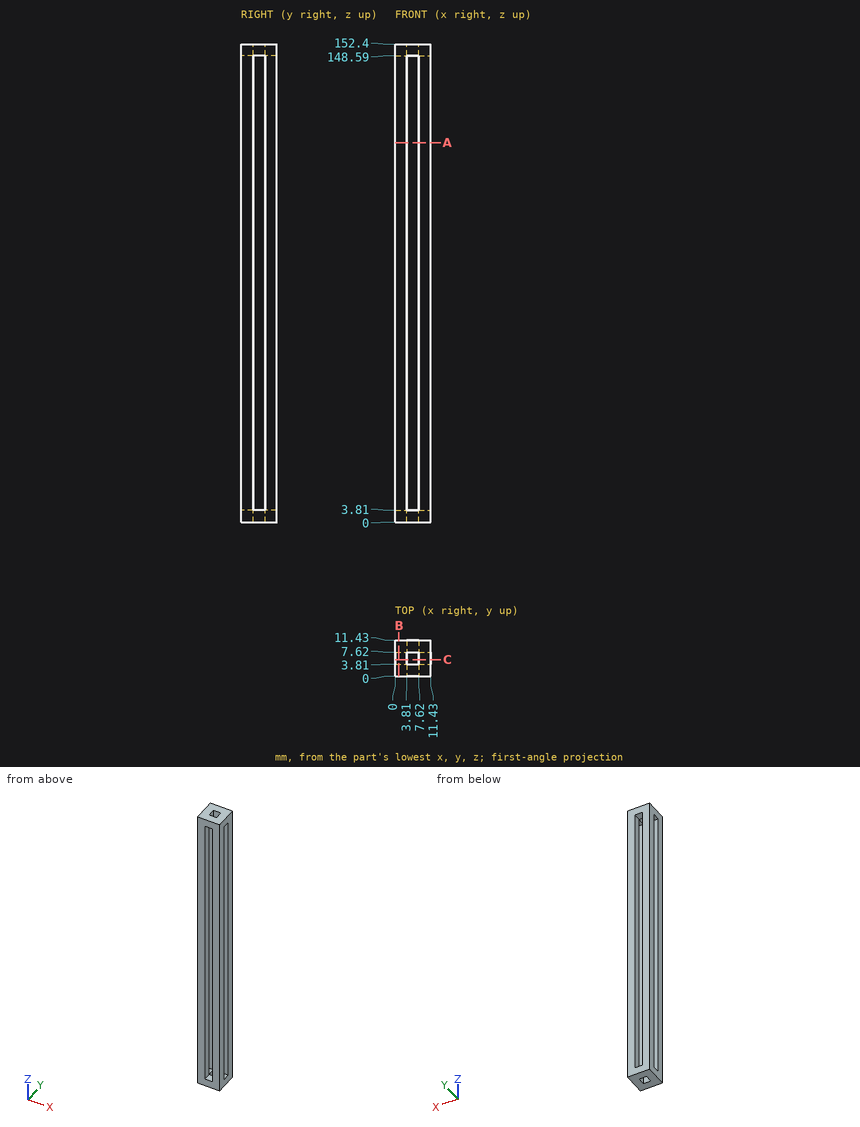
Check sheet for the drawn part. Datum: minimum x, y, z corner. Units: mm. Round coordinates to 2 decimals unless told otherwise and drop trailing zeros. Order: outer loops, then holes, each group sorted by start corner. A loop starts at its lowest first (then second) coordinate and runs counter-clockwise, first axis right, second up.
(1) Scan lines: probe 1 along X at (y, z) = (3.25, 108); probe 2 along Z at (x, y) = (7.25, 3.25). Record each from-to range of solid material in increasing order.
(2) Go/stop test with a flat-tipped pin: P1, Ø3, axis at x = 8.5, y = 5.5, coming from the -Z side. Record where the tip stops, or that it passes through.
(3) Cross-section at B-B, the plane x = 1.25. Enter the section's corners in (y, z), and give its area (3 significant figures).
(4) Cross-section at C-C, the plane y = 5.25. Enter the section's corners in (x, z).
(5) Cross-section at A-A, the plane z = 121. Enter the section's corners in (x, y), and give its area (3 significant figures).
Check sheet entries:
1. probe 1: x = 0 to 3.81, 7.62 to 11.43
1. probe 2: z = 0 to 3.81, 148.59 to 152.4
2. P1: stops at z = 0
3. outline: (0, 0) - (11.43, 0) - (11.43, 152.4) - (0, 152.4) - close; hole (3.81, 3.81) - (7.62, 3.81) - (7.62, 148.59) - (3.81, 148.59) - close
3. area: 1,190 mm2
4. outline: (0, 0) - (3.81, 0) - (3.81, 3.81) - (0, 3.81) - close; (0, 148.59) - (3.81, 148.59) - (3.81, 152.4) - (0, 152.4) - close; (7.62, 0) - (11.43, 0) - (11.43, 3.81) - (7.62, 3.81) - close; (7.62, 148.59) - (11.43, 148.59) - (11.43, 152.4) - (7.62, 152.4) - close
5. outline: (0, 0) - (3.81, 0) - (3.81, 3.81) - (0, 3.81) - close; (0, 7.62) - (3.81, 7.62) - (3.81, 11.43) - (0, 11.43) - close; (7.62, 0) - (11.43, 0) - (11.43, 3.81) - (7.62, 3.81) - close; (7.62, 7.62) - (11.43, 7.62) - (11.43, 11.43) - (7.62, 11.43) - close
5. area: 58.1 mm2
